from build123d import *

# Parameters (mm, degrees)
SKETCH1_R           = 3.96875
BOSS_EXTRUDE1_DEPTH = 140
SKETCH3_W           = 2.38125
SKETCH3_H           = 1.190625
CUT_EXTRUDE2_DEPTH  = 141.112461805
FILLET1_R           = 0.5


with BuildPart() as part:
    # Sketch1 → Boss-Extrude1 (new body)
    with BuildSketch(Plane.XY):
        Circle(SKETCH1_R)
    extrude(amount=BOSS_EXTRUDE1_DEPTH)

    # Sketch3 → Cut-Extrude2 (cut, through all)
    with BuildSketch(Plane(origin=(0, 0, 0), x_dir=(-1, 0, 0), z_dir=(0, 0, -1))):
        with Locations((0, 3.3734375)):
            Rectangle(SKETCH3_W, SKETCH3_H)
    extrude(amount=-CUT_EXTRUDE2_DEPTH, mode=Mode.SUBTRACT)

    # Fillet1
    fillet1_edges = [part.edges().sort_by_distance(p)[0] for p in [
        (0, -3.96875, 0),
        (0, -3.96875, 140),
    ]]
    fillet(fillet1_edges, radius=FILLET1_R)


solid = part.part
The listing builds one solid part. Answer for the finished solid, in the listing's coordinates (mm). Give positions to 0.01 mm unless a question says otherwise; leave off trailing zeros. Write each loop counter-clockwise with the first axis right and the second up, starting at its lowest first coordinate (ties: lowest second). Pieces come first, ordered by that corner, then holes.
1) Find the intervals of material crossed by L1, parallel to X at y = 3.5, z = 37.5; L2, parallel to Y at x = -0.25, z = 88.5; L3, parallel to X at y = 3, z = 40, in increasing order.
2) Section A-A (x = 0) is taken. Write down the section's boundary in (y, z).
3) Section B-B (z = 105) is taken. Write down the section's boundary in (x, y).
4) For a pull along X with two mould halves and no side action, classify faces 1 (the face through (0, 2.778, 69)), 2 (the face through (-0.158, -3.966, 69.027)), 3 (the face through (0, 0, 0)) as pulls with the +X half, pulls with the -X half, needs draft (parallel to the pull), parting line crosses it, or undercut.
5) Given P1, Ø0.7, axis at x = 0.5, z = 95, coming from the +Y side; P2, Ø4, axis at x = -3, z = 20.5, coming from the -Y side; P3, Ø1, axis at y = -2, z = 39.5, coming from the -X side, each flat-ended and moving along its own axis, determine where each tip first touches the part or whether it passes through.
Response:
1. L1: x = -1.87 to -1.19, 1.19 to 1.87
1. L2: y = -3.96 to 2.78
1. L3: x = -2.6 to -1.19, 1.19 to 2.6
2. outline: (-3.97, 0.5) arc R0.5 ccw to (-3.47, 0) - (2.78, 0) - (2.78, 140) - (-3.47, 140) arc R0.5 ccw to (-3.97, 139.5) - close
3. outline: (-1.19, 2.78) - (-1.19, 3.79) arc R3.97 ccw (long way) to (1.19, 3.79) - (1.19, 2.78) - close
4. face 1: undercut
4. face 2: parting line crosses it
4. face 3: needs draft
5. P1: stops at y = 2.78
5. P2: stops at y = -3.84
5. P3: stops at x = -3.67
